from build123d import *

# Parameters (mm, degrees)
F0_W      = 100
F0_H      = 100
F1_DEPTH  = 10
F2_W      = 10
F2_H      = 10
F3_DEPTH  = 10
F4_W      = 10
F4_H      = 10
F5_DEPTH  = 25
F6_W      = 10
F6_H      = 10
F7_DEPTH  = 10
F8_W      = 10
F8_H      = 10
F9_DEPTH  = 10
F10_W     = 10
F10_H     = 10
F11_DEPTH = 10
F12_W     = 10
F12_H     = 10
F13_DEPTH = 10
F14_W     = 10
F14_H     = 10
F15_DEPTH = 20
F16_W     = 10
F16_H     = 10
F17_DEPTH = 10
F18_W     = 10
F18_H     = 10
F19_DEPTH = 10
F20_W     = 10
F20_H     = 10
F21_DEPTH = 10
F22_W     = 10
F22_H     = 10
F23_DEPTH = 10
F24_W     = 10
F24_H     = 10
F25_DEPTH = 10


with BuildPart() as f1:
    # F0 (on Right) → F1 (new body)
    with BuildSketch(Plane.YZ):
        with Locations((23.273025, 4.85197)):
            Rectangle(F0_W, F0_H)
    extrude(amount=F1_DEPTH)

    # F2 (on face) → F3 (cut)
    with BuildSketch(Plane.YZ.offset(10)):
        with Locations((-21.726975, 49.85197)):
            Rectangle(F2_W, F2_H)
    extrude(amount=-F3_DEPTH, mode=Mode.SUBTRACT)

    # F4 (on face) → F5 (cut)
    with BuildSketch(Plane.YZ.offset(10)):
        with Locations((-21.726975, 19.85197)):
            Rectangle(F4_W, F4_H)
    extrude(amount=-F5_DEPTH, mode=Mode.SUBTRACT)

    # F6 (on face) → F7 (cut)
    with BuildSketch(Plane.YZ.offset(10)):
        with Locations((-21.726975, -10.14803)):
            Rectangle(F6_W, F6_H)
    extrude(amount=-F7_DEPTH, mode=Mode.SUBTRACT)

    # F8 (on face) → F9 (cut)
    with BuildSketch(Plane.YZ.offset(10)):
        with Locations((-21.726975, -40.14803)):
            Rectangle(F8_W, F8_H)
    extrude(amount=-F9_DEPTH, mode=Mode.SUBTRACT)

    # F10 (on face) → F11 (cut)
    with BuildSketch(Plane.YZ.offset(10)):
        with Locations((8.273025, -40.14803)):
            Rectangle(F10_W, F10_H)
    extrude(amount=-F11_DEPTH, mode=Mode.SUBTRACT)

    # F12 (on face) → F13 (cut)
    with BuildSketch(Plane.YZ.offset(10)):
        with Locations((38.273025, -40.14803)):
            Rectangle(F12_W, F12_H)
    extrude(amount=-F13_DEPTH, mode=Mode.SUBTRACT)

    # F14 (on face) → F15 (cut)
    with BuildSketch(Plane.YZ.offset(10)):
        with Locations((68.273025, -40.14803)):
            Rectangle(F14_W, F14_H)
    extrude(amount=-F15_DEPTH, mode=Mode.SUBTRACT)

    # F16 (on face) → F17 (cut)
    with BuildSketch(Plane.YZ.offset(10)):
        with Locations((68.273025, -10.14803)):
            Rectangle(F16_W, F16_H)
    extrude(amount=-F17_DEPTH, mode=Mode.SUBTRACT)

    # F18 (on face) → F19 (cut)
    with BuildSketch(Plane.YZ.offset(10)):
        with Locations((68.273025, 19.85197)):
            Rectangle(F18_W, F18_H)
    extrude(amount=-F19_DEPTH, mode=Mode.SUBTRACT)

    # F20 (on face) → F21 (cut)
    with BuildSketch(Plane.YZ.offset(10)):
        with Locations((68.273025, 49.85197)):
            Rectangle(F20_W, F20_H)
    extrude(amount=-F21_DEPTH, mode=Mode.SUBTRACT)

    # F22 (on face) → F23 (cut)
    with BuildSketch(Plane.YZ.offset(10)):
        with Locations((38.273025, 49.85197)):
            Rectangle(F22_W, F22_H)
    extrude(amount=-F23_DEPTH, mode=Mode.SUBTRACT)

    # F24 (on face) → F25 (cut)
    with BuildSketch(Plane.YZ.offset(10)):
        with Locations((8.273025, 49.85197)):
            Rectangle(F24_W, F24_H)
    extrude(amount=-F25_DEPTH, mode=Mode.SUBTRACT)


solid = f1.part
Source: CAD feature listing. Evaluate the final solid. Frame: model axes, mm. A direction names the side the tool comes from. Coordinates: 2 decimals unless noted, no trailing zeros. Loops run counter-clockwise (first coordinate to the right, second up) from the corner with the lowest first, then second, coordinate; pieces in that order, holes last. Notation, with made-up numbers: (22.5, 46) -> (42.5, 46) arc R10 cw to (42.5, 57) -> close; hole circle Ø8 at (2, 61). An arc over 180 degrees is marked (long way). Answer in a Markdown table with one row per item. Add a question column.
Q1. Contact query for flat-ended pins moving along their axis: pin 1 Ø5 at (x, z) = (7.5, -40.5) entering from +Y; pin 2 Ø5 at (x, z) = (7.5, -40) entering from -Y; pin 3 Ø4 at (x, y) = (8.5, 35.5) entering from +Z. Output: stop coordinate, or through.
Q2. Reachability of faces 4 (the face through (5, -22, 24.852)), 5 (the face through (5, 3.273, -40)), 6 (the face through (5, 68, 24.852)), 7 (the face through (5, 68, -35.148)), 8 (the face through (5, 13.273, 50)) from +Z, -Z, +X, -X, +Y, -Y: full face, straight path, thin tool, end or side. Return the list, or none.
Q3. Section B-B on z = 16. Return the cut outline in (x, y).
Q4. Pull-direction query (Z, two-part tool) for faces 1 (the face through (5, 33.273, 50)), 2 (the face through (5, -22, 14.852)), 3 (the face through (5, -22, -35.148)); classes: pulls with the +Z half, pulls with the -Z half, needs draft (parallel to the pull), parting line crosses it, or undercut.
Q5. Section A-A on y = 41. Return the cut outline in (x, z).
Q6. Ray query, line 1 along Y through (x, z) = (4.75, 45.5); line 2 along Z through (x, y) = (1.75, 9.5); line 3 along Y through (x, z) = (4.5, 22). Return the intervals inside material, ascending.
Computed values:
| question | item | result |
|---|---|---|
| 1 | pin 1 | stops at y = 63.27 |
| 1 | pin 2 | stops at y = -16.73 |
| 1 | pin 3 | stops at z = 44.85 |
| 2 | face 4 | +X, -X, -Y |
| 2 | face 5 | -Z, +X, -X |
| 2 | face 6 | +X, -X, +Y |
| 2 | face 7 | -Z, +X, -X, +Y |
| 2 | face 8 | +Z, +X, -X |
| 3 | outline | (0, -16.73) -> (10, -16.73) -> (10, 63.27) -> (0, 63.27) -> close |
| 4 | face 1 | needs draft |
| 4 | face 2 | undercut |
| 4 | face 3 | pulls with the -Z half |
| 5 | outline | (0, -35.15) -> (10, -35.15) -> (10, 44.85) -> (0, 44.85) -> close |
| 6 | line 1 | y = -16.73 to 3.27, 13.27 to 33.27, 43.27 to 63.27 |
| 6 | line 2 | z = -35.15 to 44.85 |
| 6 | line 3 | y = -16.73 to 63.27 |
